from build123d import *

# Parameters (mm, degrees)
BOSS_EXTRUDE1_DEPTH    = 12.7
F_10_CLEARANCE_HOLE1_D = 4.9784


with BuildPart() as part:
    # Sketch4 → Boss-Extrude1 (new body)
    with BuildSketch(Plane(origin=(0, 0, 0), x_dir=(1, 0, 0), z_dir=(0, 1, 0))):
        Polygon((-71.608792588, 6.232898137), (-71.608792588, 25.282898137), (-52.558792588, 25.282898137), (-52.558792588, -12.817101863), (-71.608792588, -12.817101863), align=None)
    extrude(amount=BOSS_EXTRUDE1_DEPTH)

    # #10 Clearance Hole1 (through all)
    with Locations(Plane(origin=(0, 12.7, 0), x_dir=(1, 0, 0), z_dir=(0, 1, 0))):
        with Locations((-61.333792588, 18.932898137), (-61.333792588, -6.467101863)):
            Hole(F_10_CLEARANCE_HOLE1_D / 2)


solid = part.part
Work out the finished part from the listing and answer in its coordinate system (mm). Round coordinates to 2 decimals unless told otherwise and drop trailing zeros. Write each loop counter-clockwise with the first axis right and the second up, starting at its lowest first coordinate (ties: lowest second). Pieces come first, ordered by that corner, then holes. Notation, with made-up numbers: (55.5, 68.25) - (114.5, 68.25) arc R20 ccw to (114.5, 87.25) - close; hole circle Ø2 at (33, 64). An arc over 180 degrees is marked (long way). Answer in a Markdown table with one row per item. Add a question column.
1. A cutting plane is placed at C-C, the plane y = 5.25. Determine the outline of the cut face in (x, z), and give its area (3 significant figures).
2. A cutting plane is placed at D-D, the plane z = -18. Determine the outline of the cut face in (x, y).
3. A cutting plane is placed at B-B, the plane x = -62.5. Determine the outline of the cut face in (y, z), and give its area (3 significant figures).
4. The mould has two halves that part along Z. Classify faces 1 (the flat face through (-71.609, 6, -6)), 2 (the cylindrical face through (-63.633, 6.261, 7.42)), 3 (the cylindrical face through (-63.633, 6.261, -17.98)), 4 (the flat face through (-62, 6, 12.817)): +Z half, -Z half, draft (parallel to the pull), parting line (faces both ways), or undercut.
5. Given pin 1 (2 mm diameter, centred on x = -60.5, z = -13.5, fed in from -Y), flat-ended and moving along its own axis, determine where the tip first touches the part or whether it passes through.
6. A cutting plane is placed at A-A, the plane z = 8.5. Determine the outline of the cut face in (x, y).
7. Find the intervals of material crossed by line 1 along Z through (x, y) = (-59.5, 4.5); line 2 along Z through (x, y) = (-60.75, 11.5); line 3 along X through (y, z) = (6.25, -18), in increasing order. Write a range as from..to.
Worked out:
| question | item | result |
|---|---|---|
| 1 | outline | (-71.61, -25.28) - (-52.56, -25.28) - (-52.56, 12.82) - (-71.61, 12.82) - close; hole circle Ø4.98 at (-61.33, -18.93); hole circle Ø4.98 at (-61.33, 6.47) |
| 1 | area | 687 mm^2 |
| 2 | outline | (-71.61, 0) - (-63.64, 0) - (-63.64, 12.7) - (-71.61, 12.7) - close; (-59.03, 0) - (-52.56, 0) - (-52.56, 12.7) - (-59.03, 12.7) - close |
| 3 | outline | (0, -25.28) - (12.7, -25.28) - (12.7, -21.13) - (0, -21.13) - close; (0, -16.73) - (12.7, -16.73) - (12.7, 4.27) - (0, 4.27) - close; (0, 8.67) - (12.7, 8.67) - (12.7, 12.82) - (0, 12.82) - close |
| 3 | area | 372 mm^2 |
| 4 | face 1 | draft |
| 4 | face 2 | undercut |
| 4 | face 3 | undercut |
| 4 | face 4 | +Z half |
| 5 | pin 1 | y = 0 |
| 6 | outline | (-71.61, 0) - (-62.77, 0) - (-62.77, 12.7) - (-71.61, 12.7) - close; (-59.9, 0) - (-52.56, 0) - (-52.56, 12.7) - (-59.9, 12.7) - close |
| 7 | line 1 | -25.28..-20.62, -17.25..4.78, 8.15..12.82 |
| 7 | line 2 | -25.28..-21.35, -16.51..4.05, 8.89..12.82 |
| 7 | line 3 | -71.61..-63.64, -59.03..-52.56 |
